Verification items for this drawing (mm, ordinates from the low corner). A direction names the side the tool comes from. Give positions to 0.01 mm unless a question says otherwise; leave off trailing zeros. Order: outer loops, then holes, each group sorted by start corner. A loop starts at its lowest first (then second) coordinate and runs counter-clockwise, first axis right, second up.
(1) Scan lines: L1, parallel to Y at x = 84, z = 42.5; L2, parallel to Z at x = 42, y = 48; L3, parallel to X at y = 19.5, z = 5. Record each from-to range of solid material in increasing order.
(2) Sectioned sample at C-C on y = 39.5. Record the cut outline in (x, z).
(3) Sectioned sample at D-D on z = 40.5. Record the cut outline in (x, y), plus the area to 3 significant figures.
(4) Sectioned sample at B-B on z = 14. Record the cut outline in (x, y), plus the area to 4 significant figures.
(5) Access from +Z, -Z, +X, -X, +Y, -Y to the whole of each face (thin tool, end or side, straight path). Record for the marked faces 1, 2 and 3.
(6) Sectioned sample at A-A on x = 65. Record the cut outline in (y, z).
(7) Gauge pin test, flat ends, axial feed: pin 1 (1 mm diameter, centred on x = 13, z = 20.5, fed in from -Y); pin 2 (12.5 mm diameter, centred on y = 17.5, z = 14.5, fed in from +X); pin 3 (12.5 mm diameter, centred on x = 77, z = 11, fed in from -Y); pin 4 (2 mm diameter, centred on x = 16, y = 43.5, fed in from +Z). Record the tip position at first contact, or that the pin passes through.
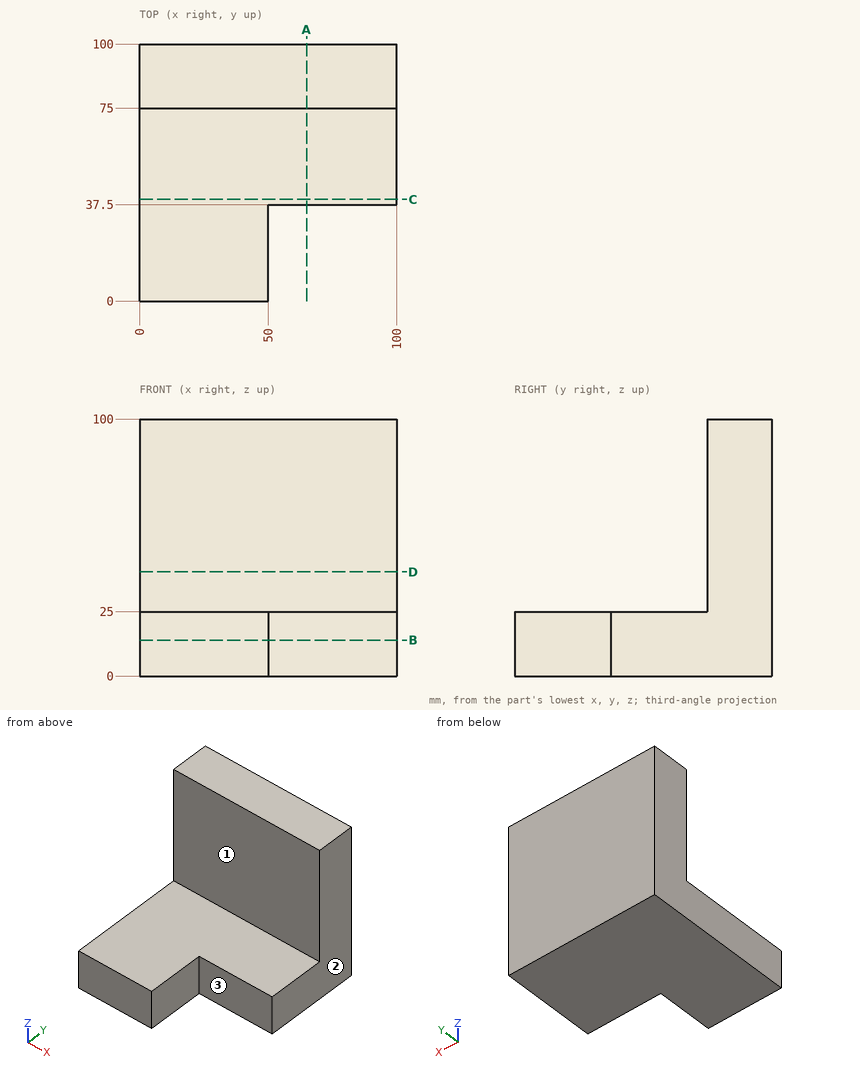
Ans:
1. L1: y = 75 to 100
1. L2: z = 0 to 25
1. L3: x = 0 to 50
2. outline: (0, 0) - (100, 0) - (100, 25) - (0, 25) - close
3. outline: (0, 75) - (100, 75) - (100, 100) - (0, 100) - close
3. area: 2,500 mm2
4. outline: (0, 0) - (50, 0) - (50, 37.5) - (100, 37.5) - (100, 100) - (0, 100) - close
4. area: 8,125 mm2
5. face 1: +Z, +X, -X, -Y
5. face 2: +Z, -Z, +X, +Y, -Y
5. face 3: +Z, -Z, +X, -Y
6. outline: (37.5, 0) - (100, 0) - (100, 100) - (75, 100) - (75, 25) - (37.5, 25) - close
7. pin 1: stops at y = 0
7. pin 2: stops at x = 50
7. pin 3: stops at y = 37.5
7. pin 4: stops at z = 25
